```python
from build123d import *

# Parameters (mm, degrees)
SKETCH_1_R      = 4.5
SKETCH_1_R_2    = 1.5
EXTRUDE_1_DEPTH = 4


with BuildPart() as part:
    # Эскиз1 → Бобышка-Вытянуть1 (new body)
    with BuildSketch(Plane(origin=(0, 0, 0), x_dir=(1, 0, 0), z_dir=(0, 1, 0))):
        with BuildLine():
            Line((-12.5, 15.852233677), (-12.5, -21.647766323))
            Line((-12.5, -21.647766323), (12.5, -21.647766323))
            Line((12.5, -21.647766323), (12.5, 15.852233677))
            ThreePointArc((12.5, 15.852233677), (0, 28.352233677), (-12.5, 15.852233677))
        make_face()
        with Locations((0, 15.852233677)):
            Circle(SKETCH_1_R, mode=Mode.SUBTRACT)
        with Locations((-7.5, -14.647766323)):
            Circle(SKETCH_1_R_2, mode=Mode.SUBTRACT)
        with Locations((7.5, -14.647766323)):
            Circle(SKETCH_1_R_2, mode=Mode.SUBTRACT)
        with Locations((-7.5, -8.147766323)):
            Circle(SKETCH_1_R_2, mode=Mode.SUBTRACT)
        with Locations((7.5, -8.147766323)):
            Circle(SKETCH_1_R_2, mode=Mode.SUBTRACT)
        with Locations((-7.5, -1.647766323)):
            Circle(SKETCH_1_R_2, mode=Mode.SUBTRACT)
        with Locations((7.5, -1.647766323)):
            Circle(SKETCH_1_R_2, mode=Mode.SUBTRACT)
        with Locations((-7.5, 4.852233677)):
            Circle(SKETCH_1_R_2, mode=Mode.SUBTRACT)
        with Locations((7.5, 4.852233677)):
            Circle(SKETCH_1_R_2, mode=Mode.SUBTRACT)
        with Locations((0, 23.102233677)):
            Circle(SKETCH_1_R_2, mode=Mode.SUBTRACT)
        with Locations((7.25, 15.852233677)):
            Circle(SKETCH_1_R_2, mode=Mode.SUBTRACT)
        with Locations((0, 8.602233677)):
            Circle(SKETCH_1_R_2, mode=Mode.SUBTRACT)
        with Locations((-7.25, 15.852233677)):
            Circle(SKETCH_1_R_2, mode=Mode.SUBTRACT)
    extrude(amount=EXTRUDE_1_DEPTH)


solid = part.part
```
Check sheet for the modelled part. Datum: model origin and axes. Units: mm. Give positions to 0.01 mm unless a question says otherwise; leave off trailing zeros. Write each loop counter-clockwise with the first axis right and the second up, starting at its lowest first coordinate (ties: lowest second). Pieces come first, ordered by that corner, then holes. Notation, with made-up numbers: (18.5, 85) - (38.5, 85) arc R7 ccw to (38.5, 95) - close; hole circle Ø6 at (45, 38.5). An arc over 180 degrees is marked (long way). Answer as a JSON object with one key per item and string values. Group by question number.
1) Release check for a two-part mould opening along X. For faces 1 (the face through (0, 0, -4)), 2 (the face through (-12.5, 2, 3)), 3 (the face through (12.5, 2, 3)), 4 (the face through (6.31, 1.97, 9.06)) record: pulls with the +X half, pulls with the -X half, needs draft (parallel to the pull), parting line crosses it, or undercut.
2) Sectioned sample at D-D (z = -21). Record the cut outline in (x, y).
3) Sectioned sample at B-B (x = -8). Record the cut outline in (y, z).
4) Thickness scan on probe 1 along X at (y, z) = (3.7, -16); probe 2 along Z at (x, y) = (0, 1.6); probe 3 along X at (y, z) = (3.75, 7.5). Record the ranges inside material, lowest first. Write a range as from..to.
5) Sectioned sample at C-C (y = 1.2). Give the number of separate pieces and of enclosed holes in the cut face, then the cut area to 3 significant figures.
6) Sectioned sample at A-A (x = 0). Record the cut outline in (y, z), then the cut area to 3 significant figures.
7) Depth check by flat-ended pin: P1, Ø7, axis at x = 0, z = -15.85, coming from the +Y side. Enter the tip coordinate at first touch or a pass-through.
Geometry results:
{
 "1": {"face 1": "needs draft", "face 2": "pulls with the -X half", "face 3": "pulls with the +X half", "face 4": "undercut"},
 "2": {"outline": "(-11.39, 0) - (11.39, 0) - (11.39, 4) - (-11.39, 4) - close"},
 "3": {"outline": "(0, -25.46) - (4, -25.46) - (4, -17.15) - (0, -17.15) - close; (0, -14.55) - (4, -14.55) - (4, -6.27) - (0, -6.27) - close; (0, -3.44) - (4, -3.44) - (4, 0.23) - (0, 0.23) - close; (0, 3.06) - (4, 3.06) - (4, 6.73) - (0, 6.73) - close; (0, 9.56) - (4, 9.56) - (4, 13.23) - (0, 13.23) - close; (0, 16.06) - (4, 16.06) - (4, 21.65) - (0, 21.65) - close"},
 "4": {"probe 1": "x = -12.5..-8.74, -5.76..-4.5, 4.5..5.76, 8.74..12.5", "probe 2": "z = -28.35..-24.6, -21.6..-20.35, -11.35..-10.1, -7.1..21.65", "probe 3": "x = -12.5..-8.85, -6.15..6.15, 8.85..12.5"},
 "5": {"separate pieces": "1", "enclosed holes": "13", "area": "1,030 mm^2"},
 "6": {"outline": "(0, -28.35) - (4, -28.35) - (4, -24.6) - (0, -24.6) - close; (0, -21.6) - (4, -21.6) - (4, -20.35) - (0, -20.35) - close; (0, -11.35) - (4, -11.35) - (4, -10.1) - (0, -10.1) - close; (0, -7.1) - (4, -7.1) - (4, 21.65) - (0, 21.65) - close", "area": "140 mm^2"},
 "7": {"P1": "passes through"}
}
